Work out the finished part from the listing and answer in its coordinate system (mm). Round coordinates to 2 decimals unless told otherwise and drop trailing zeros. Write each loop counter-clockwise with the first axis right and the second up, starting at its lowest first coordinate (ties: lowest second). Pieces come first, ordered by that corner, then holes. Notation, with made-up numbers: M -29.5,65.5 L 5.5,65.5 A21 cw 5.5,91.5 Z; hole C 24.5,15.25 d3. An arc over 180 degrees is marked long. Answer in a Markdown table with one row per item.
```python
from build123d import *

# Parameters (mm, degrees)
SKETCH_1_W      = 46
SKETCH_1_H      = 75
SKETCH_1_R      = 1.25
SKETCH_1_R_2    = 1.35
EXTRUDE_1_DEPTH = 5


with BuildPart() as part:
    # Sketch 1 → Extrude 1 (new body)
    with BuildSketch(Plane.XY):
        Rectangle(SKETCH_1_W, SKETCH_1_H)
        with Locations((-19, 32.5)):
            Circle(SKETCH_1_R, mode=Mode.SUBTRACT)
        with Locations((-15.5, -30)):
            Circle(SKETCH_1_R_2, mode=Mode.SUBTRACT)
        with Locations((-15.5, 0)):
            Circle(SKETCH_1_R_2, mode=Mode.SUBTRACT)
        with Locations(Location((15.5, -30, 0), (0, 0, 180))):
            Circle(SKETCH_1_R_2, mode=Mode.SUBTRACT)
        with Locations(Location((15.5, 0, 0), (0, 0, 180))):
            Circle(SKETCH_1_R_2, mode=Mode.SUBTRACT)
        with Locations(Location((19, 32.5, 0), (0, 0, 180))):
            Circle(SKETCH_1_R, mode=Mode.SUBTRACT)
        with Locations((-19, 12.5)):
            Circle(SKETCH_1_R, mode=Mode.SUBTRACT)
        with Locations(Location((19, 12.5, 0), (0, 0, 180))):
            Circle(SKETCH_1_R, mode=Mode.SUBTRACT)
    extrude(amount=EXTRUDE_1_DEPTH)


solid = part.part
```
1. Consider line 1 along Y through (x, z) = (19, 1.4); line 2 along Y through (x, z) = (-15.5, 3.9). Determine where each line is inside the solid, lowest interval first. Write a range as from..to.
Calculated:
| item | result |
|---|---|
| line 1 | y = -37.5..11.25, 13.75..31.25, 33.75..37.5 |
| line 2 | y = -37.5..-31.35, -28.65..-1.35, 1.35..37.5 |
2. The part is cut by section A-A (y = 12.5). Determine the outline of the cut face in (x, z).
Calculated:
| item | result |
|---|---|
| outline | M -23,0 L -20.25,0 L -20.25,5 L -23,5 Z; M -17.75,0 L 17.75,0 L 17.75,5 L -17.75,5 Z; M 20.25,0 L 23,0 L 23,5 L 20.25,5 Z |
3. Determine the mould class of faces 1 (the flat face through (23, -1, 2)), 2 (the cylindrical face through (16.57, 0.82, 2.46)), 3 (the flat face through (0, -37.5, 2)) for opening direction X: released by +X, released by -X, zero draft, split by the parting line, or undercut.
Calculated:
| item | result |
|---|---|
| face 1 | released by +X |
| face 2 | undercut |
| face 3 | zero draft |
4. The part is cut by section B-B (x = 15.5). Determine the outline of the cut face in (y, z).
Calculated:
| item | result |
|---|---|
| outline | M -37.5,0 L -31.35,0 L -31.35,5 L -37.5,5 Z; M -28.65,0 L -1.35,0 L -1.35,5 L -28.65,5 Z; M 1.35,0 L 37.5,0 L 37.5,5 L 1.35,5 Z |
